from build123d import *

# Parameters (mm, degrees)
SKETCH1_W                = 42.6
SKETCH1_H                = 30.01865285
SKETCH1_W_2              = 38.6
SKETCH1_H_2              = 27.2
BOSS_EXTRUDE1_DEPTH      = 101.9
BOSS_EXTRUDE2_DEPTH      = 13.6
BOSS_EXTRUDE2_DEPTH_BACK = 13.6
SKETCH4_W                = 2
SKETCH4_H                = 34.93
BOSS_EXTRUDE3_DEPTH      = 101.9
SKETCH5_R                = 8
CUT_EXTRUDE1_DEPTH       = 2
CUT_EXTRUDE2_REACH       = 38.339
SKETCH6_W                = 10
SKETCH6_H                = 2
SKETCH7_W                = 12
SKETCH7_H                = 4
SKETCH7_W_2              = 10
SKETCH7_H_2              = 2
CUT_EXTRUDE3_DEPTH       = 0.6
SKETCH8_W                = 2
SKETCH8_H                = 9
CUT_EXTRUDE4_DEPTH       = 70


with BuildPart() as part:
    # Sketch1 → Boss-Extrude1 (new body)
    with BuildSketch(Plane.XY):
        Rectangle(SKETCH1_W, SKETCH1_H)
        Rectangle(SKETCH1_W_2, SKETCH1_H_2, mode=Mode.SUBTRACT)
    extrude(amount=BOSS_EXTRUDE1_DEPTH)

    # Sketch3 → Boss-Extrude2 (add, two sides)
    with BuildSketch(Plane(origin=(0, 0, 0), x_dir=(0, 0, -1), z_dir=(1, 0, 0))) as boss_extrude2_sk:
        with BuildLine():
            Line((-12, 15.009326425), (0, 15.009326425))
            Line((0, 15.009326425), (0, 49.939326425))
            Line((0, 49.939326425), (-101.9, 49.939326425))
            Line((-101.9, 49.939326425), (-101.9, 47.939326425))
            Line((-101.9, 47.939326425), (-12, 47.939326425))
            Line((-12, 47.939326425), (-12, 45.640749382))
            ThreePointArc((-12, 45.640749382), (-11.256013823, 43.317309263), (-9.300813008, 41.85817281))
            ThreePointArc((-9.300813008, 41.85817281), (-3.719128817, 33.446145776), (-10.388349515, 25.867300712))
            ThreePointArc((-10.388349515, 25.867300712), (-11.545428586, 25.174874775), (-12, 23.905366805))
            Line((-12, 23.905366805), (-12, 15.009326425))
        make_face()
    extrude(amount=BOSS_EXTRUDE2_DEPTH)
    extrude(boss_extrude2_sk.sketch, amount=-BOSS_EXTRUDE2_DEPTH_BACK)

    # Sketch4 → Boss-Extrude3 (add)
    with BuildSketch(Plane(origin=(0, 0, 0), x_dir=(-1, 0, 0), z_dir=(0, 0, -1))):
        with Locations((14.6, 32.474326425)):
            Rectangle(SKETCH4_W, SKETCH4_H)
        with Locations((-14.6, 32.474326425)):
            Rectangle(SKETCH4_W, SKETCH4_H)
    extrude(amount=-BOSS_EXTRUDE3_DEPTH)

    # Sketch5 → Cut-Extrude1 (cut)
    with BuildSketch(Plane(origin=(0, 49.939326425, 0), x_dir=(1, 0, 0), z_dir=(0, 1, 0))):
        with Locations((0, -50.788349515)):
            Circle(SKETCH5_R)
    extrude(amount=-CUT_EXTRUDE1_DEPTH, mode=Mode.SUBTRACT)

    # Sketch6 → Cut-Extrude2 (cut, up to next)
    with BuildSketch(Plane.XZ.offset(-13.6), mode=Mode.PRIVATE) as cut_extrude2_sk1:
        with Locations((0, 98.9)):
            Rectangle(SKETCH6_W, SKETCH6_H)
    cut_extrude2_tool1 = extrude(cut_extrude2_sk1.sketch, amount=-CUT_EXTRUDE2_REACH, mode=Mode.PRIVATE) & part.part
    add(cut_extrude2_tool1.solids().sort_by_distance((0, 13.6, 98.9))[0], mode=Mode.SUBTRACT)

    # Sketch7 → Cut-Extrude3 (cut)
    with BuildSketch(Plane.XZ.offset(-13.6)):
        with Locations((0, 98.9)):
            Rectangle(SKETCH7_W, SKETCH7_H)
        with Locations((0, 98.9)):
            Rectangle(SKETCH7_W_2, SKETCH7_H_2, mode=Mode.SUBTRACT)
    extrude(amount=-CUT_EXTRUDE3_DEPTH, mode=Mode.SUBTRACT)

    # Sketch8 → Cut-Extrude4 (cut)
    with BuildSketch(Plane.XY.offset(101.9)):
        with Locations((-14.6, 19.509326425)):
            Rectangle(SKETCH8_W, SKETCH8_H)
    extrude(amount=-CUT_EXTRUDE4_DEPTH, mode=Mode.SUBTRACT)


solid = part.part
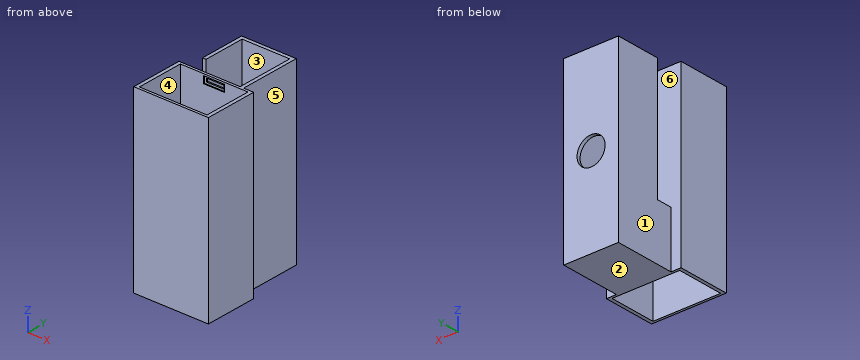
Can you work these out from the model? Positions are in its coordinate system, mm. Face numbers are marked on the shaded views. A direction names the side the tool comes from. Coordinates: 2 decimals unless noted, no trailing zeros. Loops run counter-clockwise (first coordinate to the right, second up) from the corner with the lowest first, then second, coordinate; pieces in that order, holes last. Notation, with made-up numbers: M 88,-39.75 L 117,-39.75 A8 ccw 117,-25.75 Z; hole C -32.75,-12 d11. An arc over 180 degrees is marked long. Answer as CSV lines item,"result". Start each with the question number.
1. Suppose I cut it at B-B, the plane y = 8. List the corners of the cut face in (x, z) for me, plus the area to 3 significant figures.
2. For pin 1 Ø10 at (y, z) = (36.5, 57) entering from +X; pin 2 Ø1.1 at (x, y) = (-5, 47) entering from +Z; pin 3 Ø4 at (y, z) = (43, 17) entering from -X, each with a flat end and sliding along its axis, tell me the tip position at first contact or that it passes through.
3. If I drill on probe 1 along Y at (x, z) = (-6, 17.5); probe 2 along Y at (x, z) = (-15, 87); probe 3 along X at (y, z) = (30.5, 36), over which ranges is the centre line in solid material (lowest first)? Write a range as [from, to].
4. Suppose I cut it at D-D, the plane x = 0. List the corners of the cut face in (y, z) for me, plus the area to 3 significant figures.
5. For the marked faces 4, 5 and 6, which set-ups out of +Z, -Z, +X, -X, +Y, -Y let a thin tool reach every point of the face, with its end or its side?
6. Suppose I cut it at A-A, the plane x = 10. List the corners of the cut face in (y, z) for me, plus the area to 3 significant figures.
7. Suppose I cut it at C-C, the plane z = 46.5. List the corners of the cut face in (x, y) for me.
8. Thinking about a two-plate mould opening in X: for the marked faces 1, 2 and 3, which applies, +X half, -X half, draft (parallel to the pull), parting line (faces both ways), or undercut?
Output:
1,outline,"M -21.3,0 L -19.3,0 L -19.3,101.9 L -21.3,101.9 Z; M 19.3,0 L 21.3,0 L 21.3,101.9 L 19.3,101.9 Z"
1,area,"408 mm^2"
2,pin 1,"stops at x = 15.6"
2,pin 2,"stops at z = 12"
2,pin 3,"stops at x = -15.6"
3,probe 1,"y = [-15.01, -13.6], [13.6, 15.01], [47.94, 49.94]"
3,probe 2,"y = [-15.01, -13.6], [13.6, 15.01], [24.01, 49.94]"
3,probe 3,"x = [-15.6, -13.6], [13.6, 15.6]"
4,outline,"M -15.01,0 L -13.6,0 L -13.6,101.9 L -15.01,101.9 Z; M 13.6,0 L 49.94,0 L 49.94,42.79 L 47.94,42.79 L 47.94,12 L 45.64,12 A4 ccw 41.86,9.3 A8.3 cw 25.87,10.39 A2 ccw 23.91,12 L 15.01,12 L 15.01,97.9 L 14.2,97.9 L 14.2,96.9 L 13.6,96.9 Z; M 13.6,100.9 L 14.2,100.9 L 14.2,99.9 L 15.01,99.9 L 15.01,101.9 L 13.6,101.9 Z; M 47.94,58.79 L 49.94,58.79 L 49.94,101.9 L 47.94,101.9 Z"
4,area,"739 mm^2"
5,face 4,"+Z, -Z"
5,face 5,"+Z, -Z, +X, +Y"
5,face 6,"+Z"
6,outline,"M -15.01,0 L -13.6,0 L -13.6,101.9 L -15.01,101.9 Z; M 13.6,0 L 49.94,0 L 49.94,101.9 L 47.94,101.9 L 47.94,12 L 45.64,12 A4 ccw 41.86,9.3 A8.3 cw 25.87,10.39 A2 ccw 23.91,12 L 15.01,12 L 15.01,101.9 L 13.6,101.9 Z"
6,area,"775 mm^2"
7,outline,"M -21.3,-15.01 L 21.3,-15.01 L 21.3,15.01 L 15.6,15.01 L 15.6,49.94 L 6.75,49.94 L 6.75,47.94 L 13.6,47.94 L 13.6,15.01 L -21.3,15.01 Z; M -15.6,24.01 L -13.6,24.01 L -13.6,47.94 L -6.75,47.94 L -6.75,49.94 L -15.6,49.94 Z; hole M -19.3,-13.6 L 19.3,-13.6 L 19.3,13.6 L -19.3,13.6 Z"
8,face 1,"-X half"
8,face 2,"draft"
8,face 3,"undercut"
